Read the model definition and answer for the solid it produces. Units are mm, in the model's axes. Face numbers are marked on the shaded views. A direction names the side the tool comes from. Give positions to 0.01 mm unless a question says otherwise; leave off trailing zeros. Write each loop counter-clockwise with the first axis right and the second up, starting at its lowest first coordinate (ties: lowest second). Pieces come first, ordered by that corner, then holes. Notation, with made-up numbers: (-39, 66) -> (-20, 66) arc R17 cw to (-20, 95) -> close; hole circle Ø10 at (8.25, 22.25). An arc over 180 degrees is marked (long way). Answer as CSV lines item,"result". Start each with the question number.
1. The part is cut by section D-D, the plane z = 0. Determine the outline of the cut face in (x, y).
2. Given pin 1 (1.8 mm diameter, centred on x = 15, z = 15, fed in from -Y); pin 2 (1 mm diameter, centred on y = 4, z = 26, fed in from +X); pin 3 (4 mm diameter, centred on x = 2.5, z = -1.5, fed in from +Y); pin 4 (4 mm diameter, centred on y = 4.5, z = 2, fed in from -X), each flat-ended and moving along its own axis, determine where each tip first touches the part or whether it passes through.
3. The part is cut by section C-C, the plane x = 15. Determine the outline of the cut face in (y, z).
4. The part is cut by section A-A, the plane y = 3.5. Determine the outline of the cut face in (x, z), and give its area (3 significant figures).
5. The part is cut by section B-B, the plane z = -15. Determine the outline of the cut face in (x, y).
6. Find the intervals of material crossed by line 1 (X direction, y = 3.5, z = 15); line 2 (X direction, y = 2.5, z = 16); line 3 (Z direction, x = -16, y = -6.75), in increasing order.
7. A tool of negligible diameter and unlimited length cuts with its end or side. For the marked faces 1 and 2, from which of +Z, -Z, +X, -X, +Y, -Y can it reach the whole face along a straight path? Write none if from no direction.
from build123d import *

# Parameters (mm, degrees)
SKETCH1_R           = 44.5
BOSS_EXTRUDE1_DEPTH = 6.5
SKETCH2_R           = 32.5
BOSS_EXTRUDE2_DEPTH = 8
SKETCH3_R           = 1.5
CUT_EXTRUDE1_DEPTH  = 30
CUT_EXTRUDE2_DEPTH  = 5
SKETCH5_R           = 4.5
CUT_EXTRUDE3_DEPTH  = 9
CUT_EXTRUDE4_DEPTH  = 5


with BuildPart() as part:
    # Sketch1 → Boss-Extrude1 (new body)
    with BuildSketch(Plane(origin=(0, 0, 0), x_dir=(1, 0, 0), z_dir=(0, 1, 0))):
        with Locations(Location((0, 0, 0), (0, 0, 90))):
            Circle(SKETCH1_R)
    extrude(amount=BOSS_EXTRUDE1_DEPTH)

    # Sketch2 → Boss-Extrude2 (add)
    with BuildSketch(Plane(origin=(0, 0, 0), x_dir=(1, 0, 0), z_dir=(0, 1, 0))):
        with Locations(Location((0, 0, 0), (0, 0, 270))):
            Circle(SKETCH2_R)
    extrude(amount=-BOSS_EXTRUDE2_DEPTH)

    # Sketch3 → Cut-Extrude1 (cut, symmetric)
    with BuildSketch(Plane(origin=(0, 0, 0), x_dir=(1, 0, 0), z_dir=(0, 1, 0))):
        with Locations(Location((-15, 15, 0), (0, 0, 270))):
            Circle(SKETCH3_R)
        with Locations(Location((15, 15, 0), (0, 0, 270))):
            Circle(SKETCH3_R)
        with Locations(Location((15, -15, 0), (0, 0, 270))):
            Circle(SKETCH3_R)
        with Locations(Location((-15, -15, 0), (0, 0, 270))):
            Circle(SKETCH3_R)
    extrude(amount=CUT_EXTRUDE1_DEPTH, both=True, mode=Mode.SUBTRACT)

    # Sketch4 → Cut-Extrude2 (cut)
    with BuildSketch(Plane(origin=(0, 6.5, 0), x_dir=(1, 0, 0), z_dir=(0, 1, 0))):
        Polygon((-2, 19), (2, 19), (4.5, 4.5), (19, 2), (19, -2), (4.5, -4.5), (2, -19), (-2, -19), (-4.5, -4.5), (-19, -2), (-19, 2), (-4.5, 4.5), align=None)
    extrude(amount=-CUT_EXTRUDE2_DEPTH, mode=Mode.SUBTRACT)

    # Sketch5 → Cut-Extrude3 (cut)
    with BuildSketch(Plane(origin=(0, 6.5, 0), x_dir=(1, 0, 0), z_dir=(0, 1, 0))):
        with Locations(Location((0, 0, 0), (0, 0, 270))):
            Circle(SKETCH5_R)
    extrude(amount=-CUT_EXTRUDE3_DEPTH, mode=Mode.SUBTRACT)

    # Sketch6 → Cut-Extrude4 (cut)
    with BuildSketch(Plane(origin=(0, 6.5, 0), x_dir=(1, 0, 0), z_dir=(0, 1, 0))):
        Polygon((-6.5, -4.155172414), (-6.5, 4.155172414), (-4.155172414, 6.5), (4.155172414, 6.5), (6.5, 4.155172414), (6.5, -4.155172414), (4.155172414, -6.5), (-4.155172414, -6.5), align=None)
    extrude(amount=-CUT_EXTRUDE4_DEPTH, mode=Mode.SUBTRACT)


solid = part.part
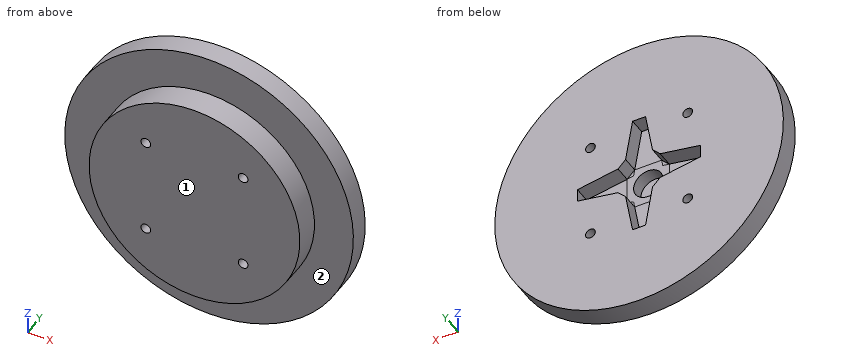
Results found:
1,outline,"(-44.5, 0) -> (-32.5, 0) -> (-32.5, -8) -> (32.5, -8) -> (32.5, 0) -> (44.5, 0) -> (44.5, 6.5) -> (19, 6.5) -> (19, 1.5) -> (4.5, 1.5) -> (4.5, -2.5) -> (-4.5, -2.5) -> (-4.5, 1.5) -> (-19, 1.5) -> (-19, 6.5) -> (-44.5, 6.5) -> close"
2,pin 1,"passes through"
2,pin 2,"stops at x = 36.47"
2,pin 3,"stops at y = 1.5"
2,pin 4,"stops at x = -44.5"
3,outline,"(-8, -28.83) -> (0, -28.83) -> (0, -41.9) -> (6.5, -41.9) -> (6.5, -16.5) -> (-8, -16.5) -> close; (-8, -13.5) -> (6.5, -13.5) -> (6.5, -2.69) -> (1.5, -2.69) -> (1.5, 2.69) -> (6.5, 2.69) -> (6.5, 13.5) -> (-8, 13.5) -> close; (-8, 16.5) -> (6.5, 16.5) -> (6.5, 41.9) -> (0, 41.9) -> (0, 28.83) -> (-8, 28.83) -> close"
4,outline,"circle Ø89 at (0, 0); hole (-19, -2) -> (-6.5, -4.16) -> (-4.16, -6.5) -> (-2, -19) -> (2, -19) -> (4.16, -6.5) -> (6.5, -4.16) -> (19, -2) -> (19, 2) -> (6.5, 4.16) -> (4.16, 6.5) -> (2, 19) -> (-2, 19) -> (-4.16, 6.5) -> (-6.5, 4.16) -> (-19, 2) -> close; hole circle Ø3 at (-15, -15); hole circle Ø3 at (-15, 15); hole circle Ø3 at (15, -15); hole circle Ø3 at (15, 15)"
4,area,"5,730 mm²"
5,outline,"(-41.9, 0) -> (-28.83, 0) -> (-28.83, -8) -> (-16.5, -8) -> (-16.5, 6.5) -> (-41.9, 6.5) -> close; (-13.5, -8) -> (13.5, -8) -> (13.5, 6.5) -> (2.69, 6.5) -> (2.69, 1.5) -> (-2.69, 1.5) -> (-2.69, 6.5) -> (-13.5, 6.5) -> close; (16.5, -8) -> (28.83, -8) -> (28.83, 0) -> (41.9, 0) -> (41.9, 6.5) -> (16.5, 6.5) -> close"
6,line 1,"x = -41.9 to -16.5, -13.5 to -2.69, 2.69 to 13.5, 16.5 to 41.9"
6,line 2,"x = -41.52 to -16.12, -13.88 to -2.52, 2.52 to 13.88, 16.12 to 41.52"
6,line 3,"z = -28.29 to -16.12, -13.88 to 13.88, 16.12 to 28.29"
7,face 1,"+Z, -Z, +X, -X, -Y"
7,face 2,"-Y"
